Check sheet for the modelled part. Datum: model origin and axes. Units: mm. A direction names the side the tool comes from. Give positions to 0.01 mm unless a question says otherwise; leave off trailing zeros. Write each loop counter-clockwise with the first axis right and the second up, starting at its lowest first coordinate (ties: lowest second). Pieces come first, ordered by that corner, then holes. Notation, with made-up numbers: M 58.5,38 L 84.5,38 A26 ccw 84.5,71 Z; hole C 53.5,12 d1. An arc over 180 degrees is marked long. Write item = value, one per line. Start each with the question number.
1) Sectioned sample at C-C, the plane z = 7.25. Record the cut outline in (x, y), then the cut area to 3 significant figures.
2) Sectioned sample at D-D, the plane z = 1.5. Record the cut outline in (x, y).
3) Sectioned sample at B-B, the plane x = 29. Record the cut outline in (y, z), then the cut area to 3 significant figures.
4) Scan lines: L1, parallel to Y at x = -29, z = 2.1; L2, parallel to Y at x = 0, z = 7; L3, parallel to X at y = 3, z = 3.5. Record each from-to range of solid material in increasing order.
5) Draft check along X on faces 5 (the face through (26, 0, 6)), 6 (the face through (0, 0, 0)), 7 (the face through (0, 0, 3)). Enter one of: pulls with the +X half, pulls with the -X half, needs draft (parallel to the pull), parting line crosses it, or undercut.
6) Gauge pin test, flat ends, axial feed: pin 1 (5.5 mm diameter, centred on x = -29, y = 13, fed in from +Z); pin 2 (1.8 mm diameter, centred on y = 5, z = 7, fed in from -X); pin 3 (3 mm diameter, centred on x = 29, y = -13, fed in from +Z); pin 4 (3 mm diameter, centred on x = 15.5, z = 5.5, fed in from -Y). Record the tip position at first contact, or that the pin passes through.
7) Sectioned sample at A-A, the plane y = 13. Record the cut outline in (x, z).
8) Set-up check for faces 1 (the face through (-26, 0, 6)), 2 (the face through (0, -11, 6)), 3 (the face through (0, 9.5, 6)), 4 (the face through (0, 11, 6)): record each of +Z, -Z, +X, -X, +Y, -Y from which the full face is reachable in a straight line by a thin tool's end or side.
Solid Edge part; units mm, degrees
sketch "Sketch1" plane through (0, 0, 0) normal (0, 0, 1) x (1, 0, 0)
  line L0 (-34, -17) -> (34, -17)
  line L1 (34, -17) -> (34, 17)
  line L2 (34, 17) -> (-34, 17)
  line L3 (-34, 17) -> (-34, -17)
  circle A0 centre (-29, -13) radius 1.7
  circle A1 centre (-29, 13) radius 1.7
  circle A2 centre (29, -13) radius 1.7
  circle A3 centre (29, 13) radius 1.7
extrude "Protrusion1" add sketch "Sketch1" along normal blind 3
sketch "Sketch2" plane through (0, 0, 3) normal (0, 0, 1) x (1, 0, 0)
  line L0 (-26, -11) -> (26, -11)
  line L1 (26, -11) -> (26, 11)
  line L2 (26, 11) -> (-26, 11)
  line L3 (-26, 11) -> (-26, -11)
  line L4 (-24.5, -9.5) -> (24.5, -9.5)
  line L5 (24.5, -9.5) -> (24.5, 9.5)
  line L6 (24.5, 9.5) -> (-24.5, 9.5)
  line L7 (-24.5, 9.5) -> (-24.5, -9.5)
extrude "ExtrudedProtrusion_2" add sketch "Sketch2" along normal blind 6
Data:
q1.outline = M -26,-11 L 26,-11 L 26,11 L -26,11 Z; hole M -24.5,-9.5 L 24.5,-9.5 L 24.5,9.5 L -24.5,9.5 Z
q1.area = 213 mm2
q2.outline = M -34,-17 L 34,-17 L 34,17 L -34,17 Z; hole C -29,-13 d3.4; hole C -29,13 d3.4; hole C 29,-13 d3.4; hole C 29,13 d3.4
q3.outline = M -17,0 L -14.7,0 L -14.7,3 L -17,3 Z; M -11.3,0 L 11.3,0 L 11.3,3 L -11.3,3 Z; M 14.7,0 L 17,0 L 17,3 L 14.7,3 Z
q3.area = 81.6 mm2
q4.L1 = -17 to -14.7, -11.3 to 11.3, 14.7 to 17
q4.L2 = -11 to -9.5, 9.5 to 11
q4.L3 = -26 to -24.5, 24.5 to 26
q5.face_5 = pulls with the +X half
q5.face_6 = needs draft
q5.face_7 = undercut
q6.pin_1 = 3
q6.pin_2 = -26
q6.pin_3 = through
q6.pin_4 = -11
q7.outline = M -34,0 L -30.7,0 L -30.7,3 L -34,3 Z; M -27.3,0 L 27.3,0 L 27.3,3 L -27.3,3 Z; M 30.7,0 L 34,0 L 34,3 L 30.7,3 Z
q8.face_1 = +Z, -X, +Y, -Y
q8.face_2 = +Z, +X, -X, -Y
q8.face_3 = +Z
q8.face_4 = +Z, +X, -X, +Y
